Source: CAD feature listing. Evaluate the final solid. Frame: model axes, mm. A direction names the side the tool comes from. Give positions to 0.01 mm unless a question says otherwise; leave off trailing zeros. Loops run counter-clockwise (first coordinate to the right, second up) from the corner with the lowest first, then second, coordinate; pieces in that order, holes last. Notation, with made-up numbers: (70, -11) -> (85, -11) arc R20 ccw to (85, 19) -> close; hole circle Ø11 at (84, 47). An arc over 180 degrees is marked (long way). Put each result on its own line as item: value.
```python
from build123d import *

# Parameters (mm, degrees)
BOSS_EXTRUDE1_DEPTH      = 90
M4_CLEARANCE_HOLE1_D     = 4.5
SKETCH4_R                = 32.5
CUT_EXTRUDE1_DEPTH       = 169.825353546
M5_CLEARANCE_HOLE1_D     = 5.5
M5_CLEARANCE_HOLE1_DEPTH = 6
CUT_EXTRUDE2_REACH       = 174.482
SKETCH7_R                = 15
FILLET1_R                = 8
FILLET2_R                = 2
FILLET3_R                = 10
TAP_DRILL_FOR_M4_TAP1_D  = 3.3


with BuildPart() as part:
    # Sketch1 → Boss-Extrude1 (new body)
    with BuildSketch(Plane.XY):
        Polygon((-53.5, 0), (53.5, 0), (53.5, 101), (47.5, 101), (47.5, 6), (-47.5, 6), (-47.5, 101), (-53.5, 101), align=None)
    extrude(amount=BOSS_EXTRUDE1_DEPTH)

    # M4 Clearance Hole1 (through all)
    with Locations(Plane(origin=(0, 6, 0), x_dir=(1, 0, 0), z_dir=(0, 1, 0))):
        with Locations((-21.25, -45), (0, -23.75), (21.25, -45), (0, -66.25)):
            Hole(M4_CLEARANCE_HOLE1_D / 2)

    # Sketch4 → Cut-Extrude1 (cut, through all)
    with BuildSketch(Plane.ZY.offset(-47.5)):
        with Locations((45, 53.5)):
            Circle(SKETCH4_R)
    extrude(amount=-CUT_EXTRUDE1_DEPTH, mode=Mode.SUBTRACT)

    # M5 Clearance Hole1
    with Locations(Plane(origin=(53.5, 0, 0), x_dir=(0, 0, -1), z_dir=(1, 0, 0))):
        with Locations((-78.587572106, 87.087572106), (-11.412427894, 87.087572106), (-11.412427894, 19.912427894), (-78.587572106, 19.912427894)):
            Hole(M5_CLEARANCE_HOLE1_D / 2, depth=M5_CLEARANCE_HOLE1_DEPTH)

    # Sketch7 → Cut-Extrude2 (cut, up to next)
    with BuildSketch(Plane.ZY.offset(53.5), mode=Mode.PRIVATE) as cut_extrude2_sk1:
        with Locations(Location((45, 53.5, 0), (0, 0, 270))):
            Circle(SKETCH7_R)
    cut_extrude2_tool1 = extrude(cut_extrude2_sk1.sketch, amount=-CUT_EXTRUDE2_REACH, mode=Mode.PRIVATE) & part.part
    add(cut_extrude2_tool1.solids().sort_by_distance((-53.5, 53.5, 45))[0], mode=Mode.SUBTRACT)

    # Fillet1
    fillet1_edges = [part.edges().sort_by_distance(p)[0] for p in [
        (53.5, 0, 45),
        (-53.5, 0, 45),
    ]]
    fillet(fillet1_edges, radius=FILLET1_R)

    # Fillet2
    fillet2_edges = [part.edges().sort_by_distance(p)[0] for p in [
        (-47.5, 6, 45),
        (47.5, 6, 45),
    ]]
    fillet(fillet2_edges, radius=FILLET2_R)

    # Fillet3
    fillet3_edges = [part.edges().sort_by_distance(p)[0] for p in [
        (-50.5, 101, 0),
        (-50.5, 101, 90),
        (50.5, 101, 90),
        (50.5, 101, 0),
    ]]
    fillet(fillet3_edges, radius=FILLET3_R)

    # Tap Drill for M4 Tap1 (through all)
    with Locations(Plane(origin=(-47.5, 0, 0), x_dir=(0, 0, -1), z_dir=(1, 0, 0))):
        with Locations((-65.506096654, 74.006096654), (-24.493903346, 74.006096654), (-24.493903346, 32.993903346), (-65.506096654, 32.993903346)):
            Hole(TAP_DRILL_FOR_M4_TAP1_D / 2)


solid = part.part
```
(1) Section B-B on x = 21.25. Return loops of the section in (y, z).
Calculated:
outline: (0, 0) -> (6, 0) -> (6, 42.75) -> (0, 42.75) -> close; (0, 47.25) -> (6, 47.25) -> (6, 90) -> (0, 90) -> close
(2) Section D-D on x = 0. Return loops of the section in (y, z).
Calculated:
outline: (0, 0) -> (6, 0) -> (6, 21.5) -> (0, 21.5) -> close; (0, 26) -> (6, 26) -> (6, 64) -> (0, 64) -> close; (0, 68.5) -> (6, 68.5) -> (6, 90) -> (0, 90) -> close
(3) Section A-A on y = 13.5. Return loops of the section in (x, z), then the cut area to 3 significant figures.
Calculated:
outline: (-53.5, 0) -> (-47.5, 0) -> (-47.5, 90) -> (-53.5, 90) -> close; (47.5, 0) -> (53.5, 0) -> (53.5, 90) -> (47.5, 90) -> close
area: 1,080 mm²
(4) Draft query along Y for faces 3 (the flat face through (1, 6, 44)), 4 (the cylindrical face through (-50.54, 34.63, 24.28)), 5 (the flat face through (-8, 5, 90)). Return one class per face: released by +Y, released by -Y, zero draft, split by the parting line, or undercut.
Calculated:
face 3: released by +Y
face 4: undercut
face 5: zero draft
(5) Reachability of faces 1 (the cylindrical face through (50.46, 84.65, 79.86)), 2 (the flat face through (-50, 101, 45)) from +Z, -Z, +X, -X, +Y, -Y: full face, straight path, thin tool, end or side. Return the list, or none.
Calculated:
face 1: +X
face 2: +Z, -Z, +X, -X, +Y
(6) First-contact query: P1, Ø3, axis at y = 74.01, z = 24.49, coming from the -X side; P2, Ø4, axis at x = -9, z = 37.5, coming from the +Y side; P3, Ø5, axis at y = 19.91, z = 11.41, coming from the +X side; P4, Ø7, axis at y = 19.91, z = 78.59, coming from the +X side. Flat tips, straight axial feed; report the tip coordinate or a pass-through.
Calculated:
P1: passes through
P2: stops at y = 6
P3: stops at x = -47.5
P4: stops at x = 53.5
(7) Section C-C on z = 45. Return loops of the section in (x, y).
Calculated:
outline: (-53.5, 8) arc R8 ccw to (-45.5, 0) -> (-23.5, 0) -> (-23.5, 6) -> (-45.5, 6) arc R2 cw to (-47.5, 8) -> (-47.5, 38.5) -> (-53.5, 38.5) -> close; (-53.5, 68.5) -> (-47.5, 68.5) -> (-47.5, 101) -> (-53.5, 101) -> close; (-19, 0) -> (19, 0) -> (19, 6) -> (-19, 6) -> close; (23.5, 0) -> (45.5, 0) arc R8 ccw to (53.5, 8) -> (53.5, 21) -> (47.5, 21) -> (47.5, 8) arc R2 cw to (45.5, 6) -> (23.5, 6) -> close; (47.5, 86) -> (53.5, 86) -> (53.5, 101) -> (47.5, 101) -> close
(8) Line query: probe 1 along Z at (x, y) = (0, 1); probe 2 along X at (y, z) = (38, 10.5); probe 3 along Z at (x, y) = (21.25, 4.25). Output: solid intervals per line, ascending. Write a range as from..to.
Calculated:
probe 1: z = 0..21.5, 26..64, 68.5..90
probe 2: x = -53.5..-47.5, 47.5..53.5
probe 3: z = 0..42.75, 47.25..90
